The listing builds one solid part. Answer for the finished solid, in the listing's coordinates (mm). A direction names the side the tool comes from. Give positions to 0.01 mm unless a question says otherwise; leave off trailing zeros. Order: outer loops, then holes, each group sorted by start corner. A loop starts at its lowest first (then second) coordinate and runs counter-clockwise, first axis right, second up. Notation, with made-up numbers: (10.25, -23.5) - (45.25, -23.5) arc R25 ccw to (45.25, 5.5) - close; hole circle Ø5 at (14.5, 9). An arc over 180 degrees is marked (long way). Answer in a Markdown table with one row per item. Add a question column.
```python
from build123d import *

# Parameters (mm, degrees)
SKETCH1_W             = 60
SKETCH1_H             = 58
BOSS_EXTRUDE1_DEPTH   = 1.6
FILLET1_R             = 2
SKETCH2_R             = 1.5
CUT_EXTRUDE1_DEPTH    = 1.6
SKETCH3_R             = 6.25
BOSS_EXTRUDE2_DEPTH   = 20
SKETCH4_W             = 5
SKETCH4_H             = 30
BOSS_EXTRUDE3_DEPTH   = 10
SKETCH5_W             = 2.54
SKETCH5_H             = 2.54
BOSS_EXTRUDE4_DEPTH   = 2
FILLET2_R             = 0.5
SKETCH6_R             = 0.5
BOSS_EXTRUDE5_DEPTH   = 7
LPATTERN1_START       = -2
LPATTERN1_DEPTH       = 2
LPATTERN1_START_2     = -9
LPATTERN1_2_OUTLINE_R = 0.5
LPATTERN1_2_DEPTH     = 7


# Read off the part's stored shape, not the designer's step: LPattern1
with BuildPart() as part:
    # Sketch1 → Boss-Extrude1 (new body)
    with BuildSketch(Plane(origin=(0, 0, 0), x_dir=(1, 0, 0), z_dir=(0, 1, 0))):
        Rectangle(SKETCH1_W, SKETCH1_H)
    extrude(amount=BOSS_EXTRUDE1_DEPTH)

    # Fillet1
    fillet1_edges = [part.edges().sort_by_distance(p)[0] for p in [
        (-30, 0.8, -29),
        (30, 0.8, -29),
        (30, 0.8, 29),
        (-30, 0.8, 29),
    ]]
    fillet(fillet1_edges, radius=FILLET1_R)

    # Sketch2 → Cut-Extrude1 (cut)
    with BuildSketch(Plane.XZ):
        with Locations(Location((-27.5, 26.5, 0), (0, 0, 270))):
            Circle(SKETCH2_R)
        with Locations(Location((-27.5, -26.5, 0), (0, 0, 90))):
            Circle(SKETCH2_R)
        with Locations(Location((27.5, -26.5, 0), (0, 0, 270))):
            Circle(SKETCH2_R)
        with Locations(Location((27.5, 26.5, 0), (0, 0, 90))):
            Circle(SKETCH2_R)
    extrude(amount=-CUT_EXTRUDE1_DEPTH, mode=Mode.SUBTRACT)

    # Sketch3 → Boss-Extrude2 (add)
    with BuildSketch(Plane.XZ):
        with Locations(Location((-15, 19, 0), (0, 0, 90))):
            Circle(SKETCH3_R)
    extrude(amount=BOSS_EXTRUDE2_DEPTH)

    # Sketch4 → Boss-Extrude3 (add)
    with BuildSketch(Plane.XZ):
        with Locations((-24, -1)):
            Rectangle(SKETCH4_W, SKETCH4_H)
    extrude(amount=BOSS_EXTRUDE3_DEPTH)

    # Sketch5 → Boss-Extrude4 (add)
    with BuildSketch(Plane.XZ):
        with Locations((25, -19)):
            Rectangle(SKETCH5_W, SKETCH5_H)
    extrude(amount=BOSS_EXTRUDE4_DEPTH)

    # Fillet2
    fillet2_edges = [part.edges().sort_by_distance(p)[0] for p in [
        (26.27, -1, -20.27),
        (26.27, -1, -17.73),
        (23.73, -1, -17.73),
        (23.73, -1, -20.27),
    ]]
    fillet(fillet2_edges, radius=FILLET2_R)

    # Sketch6 → Boss-Extrude5 (add)
    with BuildSketch(Plane.XZ.offset(2)):
        with Locations(Location((25, -19, 0), (0, 0, 90))):
            Circle(SKETCH6_R)
    extrude(amount=BOSS_EXTRUDE5_DEPTH)

    # LPattern1 outline → LPattern1 (add)
    with BuildSketch(Plane(origin=(0, 0, 0), x_dir=(1, 0, 0), z_dir=(0, 1, 0)).offset(LPATTERN1_START)):
        with BuildLine():
            Line((26.27, 15.69), (26.27, 17.23))
            ThreePointArc((26.27, 17.23), (26.123553391, 17.583553391), (25.77, 17.73))
            Line((25.77, 17.73), (24.23, 17.73))
            ThreePointArc((24.23, 17.73), (23.876446609, 17.583553391), (23.73, 17.23))
            Line((23.73, 17.23), (23.73, 15.69))
            ThreePointArc((23.73, 15.69), (23.876446609, 15.336446609), (24.23, 15.19))
            ThreePointArc((24.23, 15.19), (23.876446609, 15.043553391), (23.73, 14.69))
            Line((23.73, 14.69), (23.73, 13.15))
            ThreePointArc((23.73, 13.15), (23.876446609, 12.796446609), (24.23, 12.65))
            ThreePointArc((24.23, 12.65), (23.876446609, 12.503553391), (23.73, 12.15))
            Line((23.73, 12.15), (23.73, 10.61))
            ThreePointArc((23.73, 10.61), (23.876446609, 10.256446609), (24.23, 10.11))
            ThreePointArc((24.23, 10.11), (23.876446609, 9.963553391), (23.73, 9.61))
            Line((23.73, 9.61), (23.73, 8.07))
            ThreePointArc((23.73, 8.07), (23.876446609, 7.716446609), (24.23, 7.57))
            ThreePointArc((24.23, 7.57), (23.876446609, 7.423553391), (23.73, 7.07))
            Line((23.73, 7.07), (23.73, 5.53))
            ThreePointArc((23.73, 5.53), (23.876446609, 5.176446609), (24.23, 5.03))
            ThreePointArc((24.23, 5.03), (23.876446609, 4.883553391), (23.73, 4.53))
            Line((23.73, 4.53), (23.73, 2.99))
            ThreePointArc((23.73, 2.99), (23.876446609, 2.636446609), (24.23, 2.49))
            Line((24.23, 2.49), (25.77, 2.49))
            ThreePointArc((25.77, 2.49), (26.123553391, 2.636446609), (26.27, 2.99))
            Line((26.27, 2.99), (26.27, 4.53))
            ThreePointArc((26.27, 4.53), (26.123553391, 4.883553391), (25.77, 5.03))
            ThreePointArc((25.77, 5.03), (26.123553391, 5.176446609), (26.27, 5.53))
            Line((26.27, 5.53), (26.27, 7.07))
            ThreePointArc((26.27, 7.07), (26.123553391, 7.423553391), (25.77, 7.57))
            ThreePointArc((25.77, 7.57), (26.123553391, 7.716446609), (26.27, 8.07))
            Line((26.27, 8.07), (26.27, 9.61))
            ThreePointArc((26.27, 9.61), (26.123553391, 9.963553391), (25.77, 10.11))
            ThreePointArc((25.77, 10.11), (26.123553391, 10.256446609), (26.27, 10.61))
            Line((26.27, 10.61), (26.27, 12.15))
            ThreePointArc((26.27, 12.15), (26.123553391, 12.503553391), (25.77, 12.65))
            ThreePointArc((25.77, 12.65), (26.123553391, 12.796446609), (26.27, 13.15))
            Line((26.27, 13.15), (26.27, 14.69))
            ThreePointArc((26.27, 14.69), (26.123553391, 15.043553391), (25.77, 15.19))
            ThreePointArc((25.77, 15.19), (26.123553391, 15.336446609), (26.27, 15.69))
        make_face()
    extrude(amount=LPATTERN1_DEPTH)

    # LPattern1 2 outline → LPattern1 2 (add)
    with BuildSketch(Plane(origin=(0, 0, 0), x_dir=(1, 0, 0), z_dir=(0, 1, 0)).offset(LPATTERN1_START_2)):
        with Locations((25, 16.46)):
            Circle(LPATTERN1_2_OUTLINE_R)
        with Locations((25, 13.92)):
            Circle(LPATTERN1_2_OUTLINE_R)
        with Locations((25, 11.38)):
            Circle(LPATTERN1_2_OUTLINE_R)
        with Locations((25, 8.84)):
            Circle(LPATTERN1_2_OUTLINE_R)
        with Locations((25, 6.3)):
            Circle(LPATTERN1_2_OUTLINE_R)
        with Locations((25, 3.76)):
            Circle(LPATTERN1_2_OUTLINE_R)
    extrude(amount=LPATTERN1_2_DEPTH)


solid = part.part
```
(1) Each of these flat-tipped pins is pushed along its axis until it touches: P1, Ø0.5, axis at y = -1, z = -3.5, coming from the +X side; P2, Ø2.5, axis at x = -25, y = -3, coming from the -Z side; P3, Ø1, axis at x = 4.5, z = 12.5, coming from the -Y side; P4, Ø1.8, axis at x = 27.5, z = -26.5, coming from the +Y side. Where does it stop, or does it pass through?
(2) Find section C-C, the plane z = 10.5. Write down the section's boundary in (x, y).
(3) For faces 4 (the face through (26.27, -1, -14)), 5 (the face through (25, -1, -20.27)), 6 (the face through (23.73, -1, -6)), 7 (the face through (-15.275, -9.86, 12.756)), 8 (the face through (-26.5, -5, -1)), determine the directions among +Z, -Z, +X, -X, +Y, -Y from which every point of the face is accessible in a straight line to the end or side of a thin tool.
(4) Straight lines are drawn through the part: line 1 (X direction, y = 0.5, z = 26.5); line 2 (Y direction, x = -7.5, z = -8); line 3 (X direction, y = -9, z = -9.5). For each, find the intervals that lie inside material, in ascending order.
(5) Find section B-B, the plane x = -15. Write down the section's boundary in (y, z), plus the area to 3 significant figures.
(6) Find section D-D, the plane y = -13.25. Write down the section's boundary in (x, z), plus the area to 3 significant figures.
(7) Find section A-A, the plane y = -6. Give the number of separate pieces and of enclosed holes in the cut face, plus the area to 3 significant figures.
(8) The mould has two halves that part along Z. Classify faces 1 (the face through (28.51, 0.79, -25.39)), 2 (the face through (26.27, -1, -6)), 3 (the face through (-29.43, 0.81, -28.4)): +Z half, -Z half, draft (parallel to the pull), parting line (faces both ways), or undercut.
Answer key:
| question | item | result |
|---|---|---|
| 1 | P1 | x = 26.27 |
| 1 | P2 | z = -16 |
| 1 | P3 | y = 0 |
| 1 | P4 | through |
| 2 | outline | (-30, 0) - (-26.5, 0) - (-26.5, -10) - (-21.5, -10) - (-21.5, 0) - (30, 0) - (30, 1.6) - (-30, 1.6) - close |
| 3 | face 4 | +Z, -Z, +X, -Y |
| 3 | face 5 | -Z, +X, -X, -Y |
| 3 | face 6 | +Z, -Z, -Y |
| 3 | face 7 | -Y |
| 3 | face 8 | +Z, -Z, -X, -Y |
| 4 | line 1 | -30 to -29, -26 to 26, 29 to 30 |
| 4 | line 2 | 0 to 1.6 |
| 4 | line 3 | -26.5 to -21.5 |
| 5 | outline | (-20, 12.75) - (0, 12.75) - (0, -29) - (1.6, -29) - (1.6, 29) - (0, 29) - (0, 25.25) - (-20, 25.25) - close |
| 5 | area | 343 mm² |
| 6 | outline | circle Ø12.5 at (-15, 19) |
| 6 | area | 123 mm² |
| 7 | separate pieces | 9 |
| 7 | enclosed holes | 0 |
| 7 | area | 278 mm² |
| 8 | face 1 | undercut |
| 8 | face 2 | draft |
| 8 | face 3 | -Z half |
